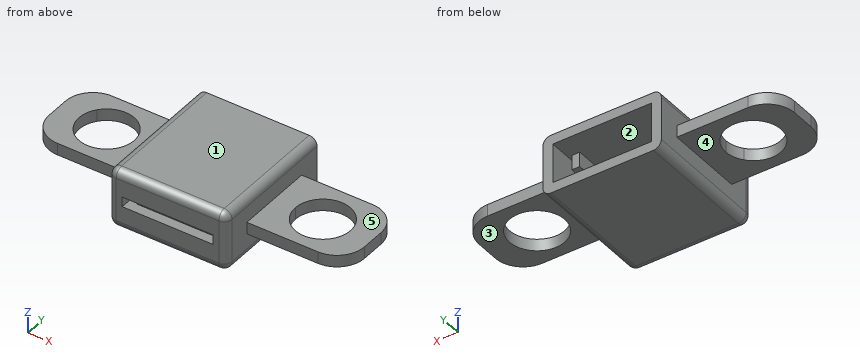
```python
from build123d import *

# Parameters (mm, degrees)
SKETCH1_W           = 30
SKETCH1_H           = 15
BOSS_EXTRUDE1_DEPTH = 33
SKETCH2_W           = 25
SKETCH2_H           = 10
CUT_EXTRUDE1_DEPTH  = 30.5
SKETCH3_W           = 23
SKETCH3_H           = 2.5
CUT_EXTRUDE2_DEPTH  = 30.5
SKETCH4_W           = 2
SKETCH4_H           = 3.75
BOSS_EXTRUDE2_DEPTH = 25
SKETCH5_W           = 2
SKETCH5_H           = 3.75
BOSS_EXTRUDE3_DEPTH = 25
SKETCH6_W           = 2
SKETCH6_H           = 3.75
BOSS_EXTRUDE4_DEPTH = 25
SKETCH7_W           = 2
SKETCH7_H           = 3.75
BOSS_EXTRUDE5_DEPTH = 25
FILLET1_R           = 2
BOSS_EXTRUDE6_DEPTH = 25
CUT_EXTRUDE3_DEPTH  = 25
FILLET2_R           = 7
FILLET3_R           = 7
BOSS_EXTRUDE7_DEPTH = 25
CUT_EXTRUDE4_DEPTH  = 25
FILLET4_R           = 7


with BuildPart() as part:
    # Sketch1 → Boss-Extrude1 (new body)
    with BuildSketch(Plane(origin=(0, 0, 0), x_dir=(1, 0, 0), z_dir=(0, 1, 0))):
        Rectangle(SKETCH1_W, SKETCH1_H)
    extrude(amount=BOSS_EXTRUDE1_DEPTH)

    # Sketch2 → Cut-Extrude1 (cut)
    with BuildSketch(Plane(origin=(0, 33, 0), x_dir=(1, 0, 0), z_dir=(0, 1, 0))):
        Rectangle(SKETCH2_W, SKETCH2_H)
    extrude(amount=-CUT_EXTRUDE1_DEPTH, mode=Mode.SUBTRACT)

    # Sketch3 → Cut-Extrude2 (cut)
    with BuildSketch(Plane(origin=(0, 2.5, 0), x_dir=(1, 0, 0), z_dir=(0, 1, 0))):
        Rectangle(SKETCH3_W, SKETCH3_H)
    extrude(amount=-CUT_EXTRUDE2_DEPTH, mode=Mode.SUBTRACT)

    # Sketch4 → Boss-Extrude2 (add)
    with BuildSketch(Plane(origin=(0, 2.5, 0), x_dir=(1, 0, 0), z_dir=(0, 1, 0))):
        with Locations((-10.5, -3.125)):
            Rectangle(SKETCH4_W, SKETCH4_H)
    extrude(amount=BOSS_EXTRUDE2_DEPTH)

    # Sketch5 → Boss-Extrude3 (add)
    with BuildSketch(Plane(origin=(0, 2.5, 0), x_dir=(1, 0, 0), z_dir=(0, 1, 0))):
        with Locations((10.5, -3.125)):
            Rectangle(SKETCH5_W, SKETCH5_H)
    extrude(amount=BOSS_EXTRUDE3_DEPTH)

    # Sketch6 → Boss-Extrude4 (add)
    with BuildSketch(Plane(origin=(0, 2.5, 0), x_dir=(1, 0, 0), z_dir=(0, 1, 0))):
        with Locations((-10.5, 3.125)):
            Rectangle(SKETCH6_W, SKETCH6_H)
    extrude(amount=BOSS_EXTRUDE4_DEPTH)

    # Sketch7 → Boss-Extrude5 (add)
    with BuildSketch(Plane(origin=(0, 2.5, 0), x_dir=(1, 0, 0), z_dir=(0, 1, 0))):
        with Locations((10.5, 3.125)):
            Rectangle(SKETCH7_W, SKETCH7_H)
    extrude(amount=BOSS_EXTRUDE5_DEPTH)

    # Fillet1
    fillet1_edges = [part.edges().sort_by_distance(p)[0] for p in [
        (0, 0, 7.5),
        (-15, 0, 0),
        (0, 0, -7.5),
        (15, 0, 0),
        (15, 16.5, 7.5),
        (-15, 16.5, 7.5),
        (-15, 16.5, -7.5),
        (15, 16.5, -7.5),
    ]]
    fillet(fillet1_edges, radius=FILLET1_R)

    # Sketch8 → Boss-Extrude6 (add)
    with BuildSketch(Plane.ZY.offset(15)):
        Polygon((1.563932113, 13.092554953), (-1.436067887, 21.547100408), (-1.436067887, 7.31982768), (1.563932113, 7.31982768), align=None)
        Polygon((-1.436067887, 27.31982768), (-1.436067887, 21.547100408), (1.563932113, 13.092554953), (1.563932113, 27.31982768), align=None)
    extrude(amount=BOSS_EXTRUDE6_DEPTH)

    # Sketch9 → Cut-Extrude3 (cut)
    with BuildSketch(Plane.XY.offset(1.563932113)):
        with BuildLine():
            ThreePointArc((-20.409219381, 17.247203185), (-25.092170791, 23.852601419), (-32.875301047, 21.620068518))
            Line((-32.875301047, 21.620068518), (-21.943137715, 12.874337852))
            ThreePointArc((-21.943137715, 12.874337852), (-20.803821147, 14.930154595), (-20.409219381, 17.247203185))
        make_face()
        with BuildLine():
            Line((-21.943137715, 12.874337852), (-32.875301047, 21.620068518))
            ThreePointArc((-32.875301047, 21.620068518), (-31.782084714, 11.781121519), (-21.943137715, 12.874337852))
        make_face()
    extrude(amount=-CUT_EXTRUDE3_DEPTH, mode=Mode.SUBTRACT)

    # Fillet2
    fillet2_edges = [part.edges().sort_by_distance(p)[0] for p in [
        (-40, 7.31982768, 0.063932113),
    ]]
    fillet(fillet2_edges, radius=FILLET2_R)

    # Fillet3
    fillet3_edges = [part.edges().sort_by_distance(p)[0] for p in [
        (-40, 27.31982768, 0.063932113),
    ]]
    fillet(fillet3_edges, radius=FILLET3_R)

    # Sketch10 → Boss-Extrude7 (add)
    with BuildSketch(Plane(origin=(15, 0, 0), x_dir=(0, 0, -1), z_dir=(1, 0, 0))):
        Polygon((1.545363578, 13.144884462), (-1.454636422, 21.599429916), (-1.454636422, 7.372157189), (1.545363578, 7.372157189), align=None)
        Polygon((-1.454636422, 27.372157189), (-1.454636422, 21.599429916), (1.545363578, 13.144884462), (1.545363578, 27.372157189), align=None)
    extrude(amount=BOSS_EXTRUDE7_DEPTH)

    # Sketch11 → Cut-Extrude4 (cut)
    with BuildSketch(Plane(origin=(0, 0, -1.545363578), x_dir=(-1, 0, 0), z_dir=(0, 0, -1))):
        with BuildLine():
            ThreePointArc((-20.397153498, 17.289879987), (-25.080104908, 23.895278222), (-32.863235164, 21.66274532))
            Line((-32.863235164, 21.66274532), (-21.931071832, 12.917014654))
            ThreePointArc((-21.931071832, 12.917014654), (-20.791755264, 14.972831397), (-20.397153498, 17.289879987))
        make_face()
        with BuildLine():
            Line((-21.931071832, 12.917014654), (-32.863235164, 21.66274532))
            ThreePointArc((-32.863235164, 21.66274532), (-31.770018831, 11.823798321), (-21.931071832, 12.917014654))
        make_face()
    extrude(amount=-CUT_EXTRUDE4_DEPTH, mode=Mode.SUBTRACT)

    # Fillet4
    fillet4_edges = [part.edges().sort_by_distance(p)[0] for p in [
        (40, 27.372157189, -0.045363578),
        (40, 7.372157189, -0.045363578),
    ]]
    fillet(fillet4_edges, radius=FILLET4_R)


solid = part.part
```
The model under review builds one solid part; all positions refer to its coordinate system, in mm. Face numbers are marked on the shaded views. A direction names the side the tool comes from. Round coordinates to 2 decimals unless told otherwise and drop trailing zeros. Loops run counter-clockwise (first coordinate to the right, second up) from the corner with the lowest first, then second, coordinate; pieces in that order, holes last. Notation, with made-up numbers: (38, 52) - (89, 52) arc R7 cw to (89, 59) - close; hole circle Ø10 at (-21.75, -1.5). An arc over 180 degrees is marked (long way). Use a Markdown table: item, result. Add a question column.
Q1. Machinability: for the marked faces 3, 4 and 5, which of the approach directions +Z, -Z, +X, -X, +Y, -Y give a long, thin tool a straight path to every point of the face, cutting with its end or side? Answer none if there is none.
Q2. Add section D-D (x = 25.5). State the section outline as (y, z) points.
Q3. For probe 1 along X at (y, z) = (5, 4.5); probe 2 along X at (y, z) = (30.5, -0.5); probe 3 along Z at (x, y) = (0.5, 16.5), list the stretches that pass through material, from the lowest coordinate up.
Q4. Add section B-B (z = -2.5). State the section outline as (x, y) points, plus the area to 3 significant figures.
Q5. Add section C-C (y = 12). State how many separate pieces and enclosed holes the cut face has, plus the area to 3 significant figures.
Q6. The part is to be moulded in two halves that separate along X. For the marked faces 1 and 2, say which applies: pulls with the +X half, pulls with the -X half, needs draft (parallel to the pull), parting line crosses it, or undercut.
Q7. Add section A-A (x = 2). State the section outline as (y, z) points, plus the area to 3 significant figures.
Q8. Insertion check: pin 1 Ø1.1 at (y, z) = (13.5, 4) entering from +X; pin 2 Ø6 at (x, y) = (-25, 21) entering from -Z; pin 3 Ø1.9 at (y, z) = (18.5, 4) entering from -X. Each pin has a flat end and moves straight along its axis. Give the tip position at first contact, or say it passes through.
Worked answers:
| question | item | result |
|---|---|---|
| 1 | face 3 | -Z, +X, +Y, -Y |
| 1 | face 4 | -Z, -X, +Y, -Y |
| 1 | face 5 | +Z, +X, +Y, -Y |
| 2 | outline | (7.37, -1.55) - (10.55, -1.55) - (10.55, 1.45) - (7.37, 1.45) - close; (24.03, -1.55) - (27.37, -1.55) - (27.37, 1.45) - (24.03, 1.45) - close |
| 3 | probe 1 | -15 to -12.5, -11.5 to -9.5, 9.5 to 11.5, 12.5 to 15 |
| 3 | probe 2 | -15 to -12.5, 12.5 to 15 |
| 3 | probe 3 | -7.5 to -5, 5 to 7.5 |
| 4 | outline | (-15, 2) arc R2 ccw to (-13, 0) - (13, 0) arc R2 ccw to (15, 2) - (15, 33) - (12.5, 33) - (12.5, 2.5) - (11.5, 2.5) - (11.5, 27.5) - (9.5, 27.5) - (9.5, 2.5) - (-9.5, 2.5) - (-9.5, 27.5) - (-11.5, 27.5) - (-11.5, 2.5) - (-12.5, 2.5) - (-12.5, 33) - (-15, 33) - close |
| 4 | area | 326 mm² |
| 5 | separate pieces | 3 |
| 5 | enclosed holes | 1 |
| 5 | area | 319 mm² |
| 6 | face 1 | needs draft |
| 6 | face 2 | undercut |
| 7 | outline | (0, -5.5) arc R2 ccw to (2, -7.5) - (33, -7.5) - (33, -5) - (2.5, -5) - (2.5, -1.25) - (0, -1.25) - close; (0, 1.25) - (2.5, 1.25) - (2.5, 5) - (33, 5) - (33, 7.5) - (2, 7.5) arc R2 ccw to (0, 5.5) - close |
| 7 | area | 182 mm² |
| 8 | pin 1 | x = 15 |
| 8 | pin 2 | z = -1.44 |
| 8 | pin 3 | x = -15 |
